Autodesk Inventor part; units mm, degrees
ref_plane "YZ Plane" through (0, 0, 0) normal (1, 0, 0) x (0, 1, 0)
ref_plane "XZ Plane" through (0, 0, 0) normal (0, 1, 0) x (-1, 0, 0)
ref_plane "XY Plane" through (0, 0, 0) normal (0, 0, 1) x (1, 0, 0)
sketch "Boceto1" plane through (0, 0, 0) normal (0, 0, 1) x (1, 0, 0)
  circle A0 centre (0, 0) radius 15
  dimension "d0" = 30
extrude "Extrusión1" add sketch "Boceto1" along normal blind 145.5
sketch "Boceto2" plane through (0, 0, 145.5) normal (0, 0, 1) x (1, 0, 0)
  circle A0 centre (0, 0) radius 12.5
  circle A1 centre (0, 0) radius 15
  dimension "d5" = 25
extrude "Extrusión2" cut sketch "Boceto2" against normal blind 10
sketch "Boceto3" plane through (0, 0, 145.5) normal (0, 0, 1) x (1, 0, 0)
  circle A0 centre (0, 0) radius 10
  dimension "d8" = 20
extrude "Extrusión3" cut sketch "Boceto3" against normal blind 145.5
sketch "Boceto4" plane through (0, 0, 145.5) normal (0, 0, 1) x (1, 0, 0)
  circle A0 centre (0, 0) radius 15
  circle A1 centre (0, 0) radius 12.5
  line L0 (-14.9345, 1.4) -> (-12.4214, 1.4)
  line L1 (-12.4214, 1.4) -> (-12.4214, -1.4)
  line L2 (-12.4214, -1.4) -> (-14.9345, -1.4)
  line L3 (-15.0786, 1.4) -> (-12.4214, -1.4) construction
  line L4 (-12.4214, 1.4) -> (-14.9469, -1.2612) construction
  line L5 (-1.4, -14.9345) -> (-1.4, -12.4214)
  line L6 (-1.4, -12.4214) -> (1.4, -12.4214)
  line L7 (1.4, -12.4214) -> (1.4, -14.9345)
  line L8 (-1.4, -15.0786) -> (1.4, -12.4214) construction
  line L9 (-1.4, -12.4214) -> (1.2612, -14.9469) construction
  line L10 (14.9345, -1.4) -> (12.4214, -1.4)
  line L11 (12.4214, -1.4) -> (12.4214, 1.4)
  line L12 (12.4214, 1.4) -> (14.9345, 1.4)
  line L13 (15.0786, -1.4) -> (12.4214, 1.4) construction
  line L14 (12.4214, -1.4) -> (14.9469, 1.2612) construction
  line L15 (1.4, 14.9345) -> (1.4, 12.4214)
  line L16 (1.4, 12.4214) -> (-1.4, 12.4214)
  line L17 (-1.4, 12.4214) -> (-1.4, 14.9345)
  line L18 (1.4, 15.0786) -> (-1.4, 12.4214) construction
  line L19 (1.4, 12.4214) -> (-1.2612, 14.9469) construction
  point P0 (-13.75, 0)
  point P1 (0, -13.75)
  point P2 (13.75, 0)
  point P3 (0, 13.75)
  dimension "d12" = 2.8
  dimension "d15" = 360
extrude "Extrusión4" add sketch "Boceto4" against normal blind 2.8 contours A0 L10 A1 L12 | L15 A1 L17 A0 | A0 L5 A1 L7 | L0 A1 L2 A0
sketch "Boceto5" plane through (0, 0, 0) normal (0, 0, -1) x (-1, 0, 0)
  circle A0 centre (0, 0) radius 12.5
  circle A1 centre (0, 0) radius 10
extrude "Extrusión5" cut sketch "Boceto5" against normal blind 133
fillet "Empalme1" radius 2.5 1 edges at (12.5, 0, 133)
sketch "Boceto6" plane through (0, 0, 0) normal (0, 0, -1) x (-1, 0, 0)
  circle A0 centre (0, 0) radius 12.5
  circle A1 centre (0, 0) radius 12.5
  circle A2 centre (0, 0) radius 10.925
  dimension "d22" = 21.85
extrude "Extrusión6" add sketch "Boceto6" against normal blind 5
sketch "Boceto7" plane through (0, 0, 0) normal (0, 0, -1) x (-1, 0, 0)
  circle A0 centre (0, 0) radius 17.5
  circle A1 centre (0, 0) radius 15
  dimension "d25" = 35
  dimension "d28" = 30
extrude "Extrusión7" add sketch "Boceto7" against normal blind 135.5
sketch "Boceto9" plane through (0, 0, 0) normal (0, 0, -1) x (-1, 0, 0)
  circle A0 centre (0, 0) radius 16.5
  dimension "d29" = 33
extrude "Extrusión8" cut sketch "Boceto9" against normal blind 135.5
sketch "Boceto10" plane through (0, 0, 0) normal (0, 0, -1) x (-1, 0, 0)
  circle A0 centre (0, 0) radius 16.5
  circle A1 centre (0, 0) radius 10.925
  dimension "d32" = 21.85
extrude "Extrusión9" add sketch "Boceto10" against normal blind 5
sketch "Boceto11" plane through (0, 0, 0) normal (0, 0, -1) x (-1, 0, 0)
  circle A0 centre (0, 0) radius 17.5
  circle A1 centre (0, 0) radius 20
  circle A2 centre (0, 0) radius 17.5
  dimension "d35" = 40
  dimension "d36" = 35
extrude "Extrusión10" add sketch "Boceto11" against normal blind 135.5
sketch "Boceto12" plane through (0, 0, 135.5) normal (0, 0, 1) x (1, 0, 0)
  circle A0 centre (0, 0) radius 17.5
  circle A1 centre (0, 0) radius 16.5
  dimension "d39" = 35
extrude "Extrusión11" cut sketch "Boceto12" against normal blind 134
sketch "Boceto13" plane through (0, 0, 145.5) normal (0, 0, 1) x (1, 0, 0)
  circle A0 centre (0, 0) radius 15.5
  circle A1 centre (0, 0) radius 17.5
  dimension "d42" = 31
extrude "Extrusión12" cut sketch "Boceto13" against normal blind 10 contours A0
sketch "Boceto14" plane through (0, 0, 135.5) normal (0, 0, 1) x (1, 0, 0)
  circle A0 centre (0, 0) radius 17.5
  circle A1 centre (0, 0) radius 15.5
  dimension "d45" = 31
extrude "Extrusión13" add sketch "Boceto14" along normal blind 10
sketch "Boceto15" plane through (0, 0, 145.5) normal (0, 0, 1) x (1, 0, 0)
  line L0 (-20, 1.375) -> (-16.4197, 1.375)
  line L1 (-16.4426, -1.375) -> (-20, -1.375)
  line L2 (-20, -1.375) -> (-20, 1.375)
  circle A0 centre (0, 0) radius 17.5
  line L3 (-16.4197, 1.375) -> (-16.4426, -1.375)
  circle A1 centre (0, 0) radius 16.5
  line L4 (-1.375, -20) -> (-1.375, -16.4197)
  line L5 (1.375, -16.4426) -> (1.375, -20)
  line L6 (1.375, -20) -> (-1.375, -20)
  line L7 (-1.375, -16.4197) -> (1.375, -16.4426)
  line L8 (20, -1.375) -> (16.4197, -1.375)
  line L9 (16.4426, 1.375) -> (20, 1.375)
  line L10 (20, 1.375) -> (20, -1.375)
  line L11 (16.4197, -1.375) -> (16.4426, 1.375)
  line L12 (1.375, 20) -> (1.375, 16.4197)
  line L13 (-1.375, 16.4426) -> (-1.375, 20)
  line L14 (-1.375, 20) -> (1.375, 20)
  line L15 (1.375, 16.4197) -> (-1.375, 16.4426)
  point P0 (-17.5, 0)
  point P1 (0, -17.5)
  point P2 (17.5, 0)
  point P3 (0, 17.5)
  dimension "d52" = 360
extrude "Extrusión14" add sketch "Boceto15" against normal blind 2.75 contours L0 A0 L1 L2 | L0 A1 L1 A0 | L0 L3 A1 | L13 L14 L12 A0 | A0 L12 A1 L13 | A1 L12 L15 | L4 A1 L5 A0 | A0 L5 L6 L4 | L4 L7 A1 | L9 L10 L8 A0 | A0 L8 A1 L9 | A1 L8 L11
sketch "Boceto16" plane through (0, 0, 0) normal (0, 0, -1) x (-1, 0, 0)
  circle A0 centre (0, 0) radius 20
  circle A1 centre (0, 0) radius 10.925
extrude "Extrusión15" cut sketch "Boceto16" against normal blind 1
sketch "Boceto17" plane through (0, 0, 1) normal (0, 0, -1) x (-1, 0, 0)
  circle A0 centre (0, 0) radius 17.5
  dimension "d58" = 35
extrude "Extrusión16" cut sketch "Boceto17" against normal blind 20
sketch "Boceto18" plane through (0, 0, 1) normal (0, 0, -1) x (-1, 0, 0)
  circle A0 centre (0, 0) radius 17.5
  circle A1 centre (0, 0) radius 10.925
  dimension "d61" = 21.85
  dimension "d62" = 35
extrude "Extrusión17" add sketch "Boceto18" against normal blind 5
sketch "Boceto19" plane through (0, 0, 1) normal (0, 0, -1) x (-1, 0, 0)
  circle A0 centre (0, 0) radius 10.925
  circle A1 centre (0, 0) radius 20
extrude "Extrusión18" cut sketch "Boceto19" against normal blind 2
thicken "Engrosado1" operation add thickness 1 both sides no extend neighbours no toward (-0.9870503, 0.1604113, 0) faces at (17.2734, -2.8072, 92.3333) (16.5137, -2.6325, 135.5)
fillet "Empalme2" radius 2 1 edges at (-16.5, 0, 134.5)
equation "\"Radio_pliegue\" = Grosor"
equation "\"Anchura_desahogo_plegado\" = Grosor"
equation "\"Profundidad_desahogo_plegado\" = 0.5 * Grosor"
equation "\"Tamaño_destalonado\" = 4 * Grosor"
equation "\"Remanente_mínimo\" = 2 * Grosor"
equation "\"Radiodetransición\" = Radio_pliegue"
equation "\"Tamaño_de_radio_de_Jacobi\" = Radio_pliegue"
equation "\"TamañoSeparación\" = Grosor"
properties part number "HERRAMIENTA_p2" material "Plástico PET"
Check sheet for the modelled part. Datum: model origin and axes. Units: mm. A direction names the side the tool comes from. Coordinates: 2 decimals unless noted, no trailing zeros. Loops run counter-clockwise (first coordinate to the right, second up) from the corner with the lowest first, then second, coordinate; pieces in that order, holes last.
1) Sectioned sample at A-A (y = 0). Record the boundary of the cut face in (x, z) (3 decimals), and give its area (3 significant figures).
2) Sectioned sample at C-C (z = 101). Record the boundary of the cut face in (x, y).
3) Release check for a two-part mould opening along X. For faces 5 (the face through (1.375, -19, 144)), 6 (the face through (19, -1.375, 144)), 7 (the face through (2.368, -10.665, 4.479)) record: released by +X, released by -X, zero draft, split by the parting line, or undercut.
4) Material ranges on probe 1 along X at (y, z) = (0, 139); probe 2 along X at (y, z) = (0, 4.9) (3 decimals), recorded low to high.
5) Access from +Z, -Z, +X, -X, +Y, -Y to the whole of each face (thin tool, end or side, straight path). Record for faces 1 (the face through (-2.018, 15.368, 140.077)), 2 (the face through (15.24, -6.32, 70.27)), 3 (the face through (1.375, 19, 144)), 4 (the face through (-19, -1.375, 144)).
6) Gauge pin test, flat ends, axial feed: pin 1 (1.3 mm diameter, centred on x = 18.5, z = 144.5, fed in from +Y) (3 decimals); pin 2 (2 mm diameter, centred on x = -10, y = 16, fed in from +Z); pin 3 (2 mm diameter, centred on y = -4.5, z = 99, fed in from +X); pin 4 (12 mm diameter, centred on y = -1.5, z = 83, fed in from -X). Record the tip position at first contact, or that the pin passes through.
Check sheet entries:
1. outline: (-20, 3) - (-10.925, 3) - (-10.925, 6) - (-16.5, 6) - (-16.5, 132.768) arc R2 cw to (-15.5, 134.5) - (-15.5, 145.5) - (-20, 145.5) - (-20, 142.75) - (-17.5, 142.75) - (-17.5, 135.5) - (-20, 135.5) - close; (10.925, 3) - (20, 3) - (20, 135.5) - (17.5, 135.5) - (17.5, 142.75) - (20, 142.75) - (20, 145.5) - (15.5, 145.5) - (15.5, 134.5) arc R2 cw to (16.5, 132.768) - (16.5, 6) - (10.925, 6) - close
1. area: 1,020 mm2
2. outline: circle Ø40 at (0, 0); hole circle Ø33 at (0, 0)
3. face 5: released by +X
3. face 6: zero draft
3. face 7: undercut
4. probe 1: x = -17.5 to -15.5, 15.5 to 17.5
4. probe 2: x = -20 to -10.925, 10.925 to 20
5. face 1: +Z
5. face 2: none
5. face 3: +Z, +X, +Y
5. face 4: +Z, -X, -Y
6. pin 1: stops at y = 1.375
6. pin 2: stops at z = 135.5
6. pin 3: stops at x = 19.69
6. pin 4: stops at x = -20
